Drawing for the job (mm, zero at the part's lowest x, y, z). Coordinates: 2 decimals unless noted, no trailing zeros. Loops run counter-clockwise (first coordinate to the right, second up) from the corner with the lowest first, then second, coordinate; pieces in that order, holes last.
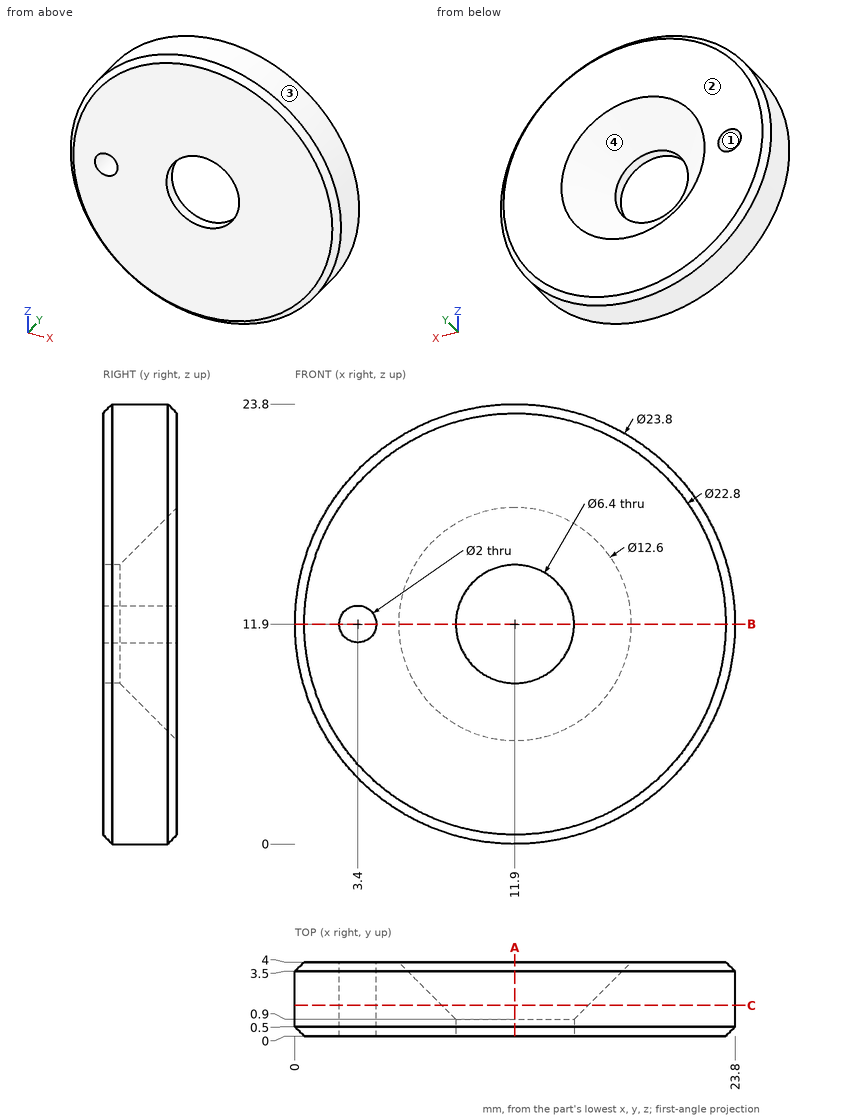
Q1. Mould opens along X. For the marked faces 1, 2, 3 and 4 say: released by +X, released by -X, zero draft, split by the parting line, or undercut.
Q2. Saw through at C-C (y = 1.65). List the corners of the cut face in (x, z).
Q3. Drop flat-ended pins along their axis: P1, Ø8.5, axis at x = 11.9, z = 11.9, coming from the -Y side; P2, Ø1.8, axis at x = 3.4, z = 11.9, coming from the -Y side; P3, Ø1, axis at x = 7, y = 3, coming from the +Z side; P4, Ø1.5, axis at y = 1, z = 16, coming from the +X side. Give the stop position or say it passes through.
Q4. Saw through at B-B (z = 11.9). List the corners of the cut face in (x, y), plus the area to 3 significant figures.
Q5. Probe line 1 (X direction, y = 0.8, z = 12); line 2 (Z direction, x = 11.9, y = 0.75); line 3 (X direction, y = 3.15, z = 12.25). List the from-to ranges inside material, lowest first.
Q6. Saw through at A-A (x = 11.9). List the corners of the cut face in (y, z).
Checked values:
1. face 1: undercut
1. face 2: zero draft
1. face 3: split by the parting line
1. face 4: undercut
2. outline: circle Ø23.8 at (11.9, 11.9); hole circle Ø2 at (3.4, 11.9); hole circle Ø7.9 at (11.9, 11.9)
3. P1: stops at y = 0
3. P2: passes through
3. P3: stops at z = 22.96
3. P4: stops at x = 23.32
4. outline: (0, 0.5) - (0.5, 0) - (2.4, 0) - (2.4, 4) - (0.5, 4) - (0, 3.5) - close; (4.4, 0) - (8.7, 0) - (8.7, 0.9) - (5.6, 4) - (4.4, 4) - close; (15.1, 0) - (23.3, 0) - (23.8, 0.5) - (23.8, 3.5) - (23.3, 4) - (18.2, 4) - (15.1, 0.9) - close
4. area: 51.5 mm2
5. line 1: x = 0 to 2.41, 4.39 to 8.7, 15.1 to 23.8
5. line 2: z = 0 to 8.7, 15.1 to 23.8
5. line 3: x = 0.01 to 2.46, 4.34 to 6.46, 17.34 to 23.79
6. outline: (0, 0.5) - (0.5, 0) - (3.5, 0) - (4, 0.5) - (4, 5.6) - (0.9, 8.7) - (0, 8.7) - close; (0, 15.1) - (0.9, 15.1) - (4, 18.2) - (4, 23.3) - (3.5, 23.8) - (0.5, 23.8) - (0, 23.3) - close
